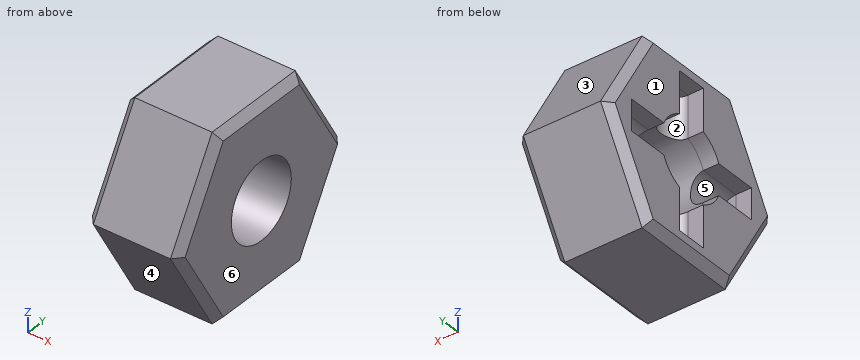
```python
from build123d import *

# Parameters (mm, degrees)
F0_R     = 2.5
F3_DEPTH = 5
F1_R     = 1
F4_DEPTH = 5
F5_DEPTH = 5
F2_R     = 1
F6_DEPTH = 5
F7_DEPTH = 5
F8_SIZE  = 0.5
F9_DEPTH = 1
F10_SIZE = 0.5


with BuildPart() as f3:
    # F0 (on Right) → F3 (new body)
    with BuildSketch(Plane.YZ):
        Polygon((3.4641016151, 6), (-3.4641016151, 6), (-6.9282032303, 0), (-3.4641016151, -6), (3.4641016151, -6), (6.9282032303, 0), align=None)
        Circle(F0_R, mode=Mode.SUBTRACT)
    extrude(amount=F3_DEPTH)

    # F1 (on Front) → F4 (cut)
    with BuildSketch(Plane.XZ):
        Circle(F1_R)
    extrude(amount=-F4_DEPTH, mode=Mode.SUBTRACT)

    # F1 (on Front) → F5 (cut)
    with BuildSketch(Plane.XZ):
        Circle(F1_R)
    extrude(amount=F5_DEPTH, mode=Mode.SUBTRACT)

    # F2 (on Top) → F6 (cut)
    with BuildSketch(Plane.XY):
        Circle(F2_R)
    extrude(amount=-F6_DEPTH, mode=Mode.SUBTRACT)

    # F2 (on Top) → F7 (cut)
    with BuildSketch(Plane.XY):
        Circle(F2_R)
    extrude(amount=F7_DEPTH, mode=Mode.SUBTRACT)

    # F8
    f8_edges = [f3.edges().sort_by_distance(p)[0] for p in [
        (5, 0, -6),
        (5, 5.196152, -3),
        (5, 5.196152, 3),
        (5, 0, 6),
        (5, -5.196152, 3),
        (5, -5.196152, -3),
    ]]
    chamfer(f8_edges, length=F8_SIZE)

    # F9 (add): a face of the model
    f9_faces = [f3.faces().sort_by_distance(p)[0] for p in [
        (0, 5.037407344, 2.9083484861),
    ]]
    extrude(f9_faces, amount=F9_DEPTH)

    # F10
    f10_edges = [f3.edges().sort_by_distance(p)[0] for p in [
        (-1, -5.196152, -3),
        (-1, 5.196152, -3),
        (-1, 0, -6),
        (-1, 0, 6),
        (-1, 5.196152, 3),
        (-1, -5.196152, 3),
    ]]
    chamfer(f10_edges, length=F10_SIZE)


solid = f3.part
```
Part model, mm, in its own coordinate system. Face numbers are marked on the shaded views. A direction names the side the tool comes from. Round coordinates to 2 decimals unless told otherwise and drop trailing zeros. Loops run counter-clockwise (first coordinate to the right, second up) from the corner with the lowest first, then second, coordinate; pieces in that order, holes last.
1. Slice it at D-D (y = -1.75). Give the cut face in (x, z).
Solutions:
outline: (-1, -5.5) - (-0.5, -6) - (4.5, -6) - (5, -5.5) - (5, -1.79) - (-1, -1.79) - close; (-1, 1.79) - (5, 1.79) - (5, 5.5) - (4.5, 6) - (-0.5, 6) - (-1, 5.5) - close
2. Two-plate mould, pull along Z, no slides. Class the marked faces 3, 4, 5 and 6: pulls with the +Z half, pulls with the -Z half, needs draft (parallel to the pull), parting line crosses it, or undercut.
Solutions:
face 3: pulls with the +Z half
face 4: pulls with the -Z half
face 5: undercut
face 6: needs draft
3. Slice it at A-A (y = 0). Give the cut face in (x, z), and give its area (3 significant figures).
Solutions:
outline: (-1, -5.5) - (-0.5, -6) - (4.5, -6) - (5, -5.5) - (5, -2.5) - (1, -2.5) - (1, -5) - (-1, -5) - close; (-1, 5) - (1, 5) - (1, 2.5) - (5, 2.5) - (5, 5.5) - (4.5, 6) - (-0.5, 6) - (-1, 5.5) - close
area: 31.5 mm2
4. 3-axis set-ups, long thin cutter, end or side, ignore diameter. For the marked faces 1 and 2: which of +Z, -Z, +X, -X, +Y, -Y reach the whole face in a straight line?
Solutions:
face 1: +Z, -Z, -X, +Y, -Y
face 2: -X
5. Flat gauge pins, fed straight in: pin 1 (0.8 mm diameter, centred on x = -0.5, z = 3, fed in from -Y); pin 2 (1.5 mm diameter, centred on x = 1.5, z = 1, fed in from -Y); pin 3 (0.8 mm diameter, centred on x = -0.5, z = -4, fed in from -Y). Where does each tip first touch, or does it go through?
Solutions:
pin 1: stops at y = -5.43
pin 2: stops at y = -6.78
pin 3: stops at y = -4.85
6. Slice it at C-C (y = 3). Give the cut face in (x, z).
Solutions:
outline: (-1, -5.5) - (-0.5, -6) - (4.5, -6) - (5, -5.5) - (5, 5.5) - (4.5, 6) - (-0.5, 6) - (-1, 5.5) - (-1, 1) - (0, 1) arc R1 cw to (0, -1) - (-1, -1) - close
7. Slice it at B-B (x = 2). Give the cut face in (y, z).
Solutions:
outline: (-6.93, 0) - (-3.46, -6) - (3.46, -6) - (6.93, 0) - (3.46, 6) - (-3.46, 6) - close; hole circle Ø5 at (0, 0)
8. Drill centre lines: line 1 along Z through (x, y) = (4.05, 0); line 2 along Z through (x, y) = (0.25, -0.25); line 3 along Y through (x, z) = (3, 2). Where is each one in solid material? Low to high.
Solutions:
line 1: z = -6 to -2.5, 2.5 to 6
line 2: z = -6 to -5, 5 to 6
line 3: y = -5.77 to -1.5, 1.5 to 5.77
